Can you work these out from the model? Positions are in its coordinate system, mm. Face numbers are marked on the shaded views. A direction names the side the tool comes from. Coordinates: 2 decimals unless noted, no trailing zeros. Order: outer loops, then holes, each group sorted by start corner. A loop starts at its lowest first (then second) coordinate and runs counter-clockwise, first axis right, second up. Notation, with made-up numbers: (-29, 17.25) -> (-4, 17.25) arc R34 ccw to (-4, 55.25) -> close; hole circle Ø3 at (9, -16.5). An arc over 180 degrees is marked (long way). Answer as CSV lines item,"result".
from build123d import *

# Parameters (mm, degrees)
F0_R     = 50.8
F1_DEPTH = 38.1
F2_R     = 42.5831
F3_DEPTH = 12.7
F4_R     = 16.51
F5_DEPTH = 25.401
F6_SIZE  = 1.27
F7_R     = 2.9972
F8_DEPTH = 25.401


with BuildPart() as f1:
    # F0 (on Top) → F1 (new body)
    with BuildSketch(Plane.XY):
        Circle(F0_R)
    extrude(amount=F1_DEPTH)

    # F2 (on face) → F3 (cut)
    with BuildSketch(Plane.XY.offset(38.1)):
        Circle(F2_R)
    extrude(amount=-F3_DEPTH, mode=Mode.SUBTRACT)

    # F4 (on face) → F5 (cut, through all)
    with BuildSketch(Plane.XY.offset(25.4)):
        Circle(F4_R)
    extrude(amount=-F5_DEPTH, mode=Mode.SUBTRACT)

    # F6
    f6_edges = [f1.edges().sort_by_distance(p)[0] for p in [
        (-42.5831, 0, 38.1),
        (-16.51, 0, 25.4),
        (-50.8, 0, 38.1),
        (-50.8, 0, 0),
    ]]
    chamfer(f6_edges, length=F6_SIZE)

    # F7 (on face) → F8 (cut, through all)
    with BuildSketch(Plane.XY.offset(25.4)):
        with Locations((35.56, 0)):
            Circle(F7_R)
        with Locations((-35.56, 0)):
            Circle(F7_R)
    extrude(amount=-F8_DEPTH, mode=Mode.SUBTRACT)


solid = f1.part
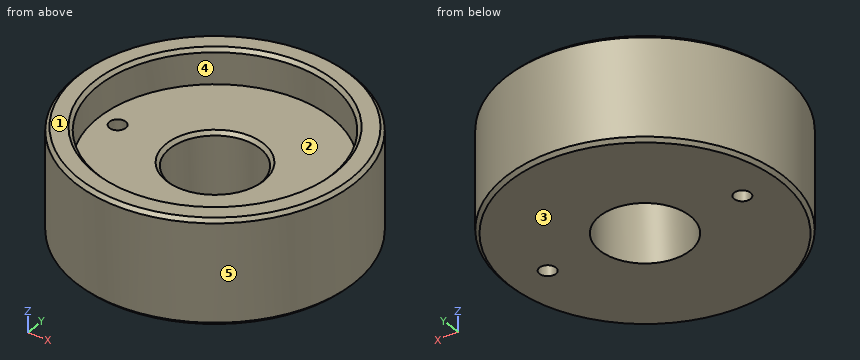
Q1. If I drill on line 1 (Y direction, x = 0, z = 29.75); line 2 (Y direction, x = 35.56, z = 8.5); line 3 (Z direction, x = 20.5, y = 26), over which ranges is the centre line in solid material (lowest first)?
Solution:
line 1,"-50.8 to -42.58, 42.58 to 50.8"
line 2,"-36.28 to -3, 3 to 36.28"
line 3,"0 to 25.4"
Q2. Imagine slicing it at B-B (y = 0). List the corners of the cut face in (x, z) for me.
Solution:
outline,"(-50.8, 1.27) -> (-49.53, 0) -> (-38.56, 0) -> (-38.56, 25.4) -> (-42.58, 25.4) -> (-42.58, 36.83) -> (-43.85, 38.1) -> (-49.53, 38.1) -> (-50.8, 36.83) -> close; (-32.56, 0) -> (-16.51, 0) -> (-16.51, 24.13) -> (-17.78, 25.4) -> (-32.56, 25.4) -> close; (16.51, 0) -> (32.56, 0) -> (32.56, 25.4) -> (17.78, 25.4) -> (16.51, 24.13) -> close; (38.56, 0) -> (49.53, 0) -> (50.8, 1.27) -> (50.8, 36.83) -> (49.53, 38.1) -> (43.85, 38.1) -> (42.58, 36.83) -> (42.58, 25.4) -> (38.56, 25.4) -> close"
Q3. Imagine slicing it at A-A (x = 0). List the corners of the cut face in (y, z) for me, and give its area (3 significant figures).
Solution:
outline,"(-50.8, 1.27) -> (-49.53, 0) -> (-16.51, 0) -> (-16.51, 24.13) -> (-17.78, 25.4) -> (-42.58, 25.4) -> (-42.58, 36.83) -> (-43.85, 38.1) -> (-49.53, 38.1) -> (-50.8, 36.83) -> close; (16.51, 0) -> (49.53, 0) -> (50.8, 1.27) -> (50.8, 36.83) -> (49.53, 38.1) -> (43.85, 38.1) -> (42.58, 36.83) -> (42.58, 25.4) -> (17.78, 25.4) -> (16.51, 24.13) -> close"
area,"1,940 mm2"
Q4. We'd pull the mould along Y, two halves only. Please class the marked faces 3, 4 and 5: pulls with the +Y half, pulls with the -Y half, needs draft (parallel to the pull), parting line crosses it, or undercut.
Solution:
face 3,"needs draft"
face 4,"undercut"
face 5,"parting line crosses it"
Q5. Imagine slicing it at C-C (z = 27). List the corners of the cut face in (x, y) for me, and give its area (3 significant figures).
Solution:
outline,"circle Ø101.6 at (0, 0); hole circle Ø85.17 at (0, 0)"
area,"2,410 mm2"
Q6. Imagine slicing it at D-D (z = 3). List the corners of the cut face in (x, y) for me.
Solution:
outline,"circle Ø101.6 at (0, 0); hole circle Ø5.99 at (-35.56, 0); hole circle Ø33.02 at (0, 0); hole circle Ø5.99 at (35.56, 0)"
Q7. For P1, Ø12, axis at x = 13.5, z = 11, coming from the -Y side; P2, Ø3, axis at y = -21.5, z = 6, coming from the -X side; P3, Ø5, axis at y = -27, z = 22, coming from the +X side, each with a flat end and sliding along its axis, tell me the tip position at first contact or that it passes through.
Solution:
P1,"y = -50.24"
P2,"x = -46.7"
P3,"x = 44.5"
Q8. Which directions (+Z, -Z, +X, -X, +Y, -Y) give clear straight access to the entire face, cutting with the end or side of a thin tool? Please do the marked faces 1 and 2.
Solution:
face 1,"+Z, +X, -X, +Y, -Y"
face 2,"+Z"
